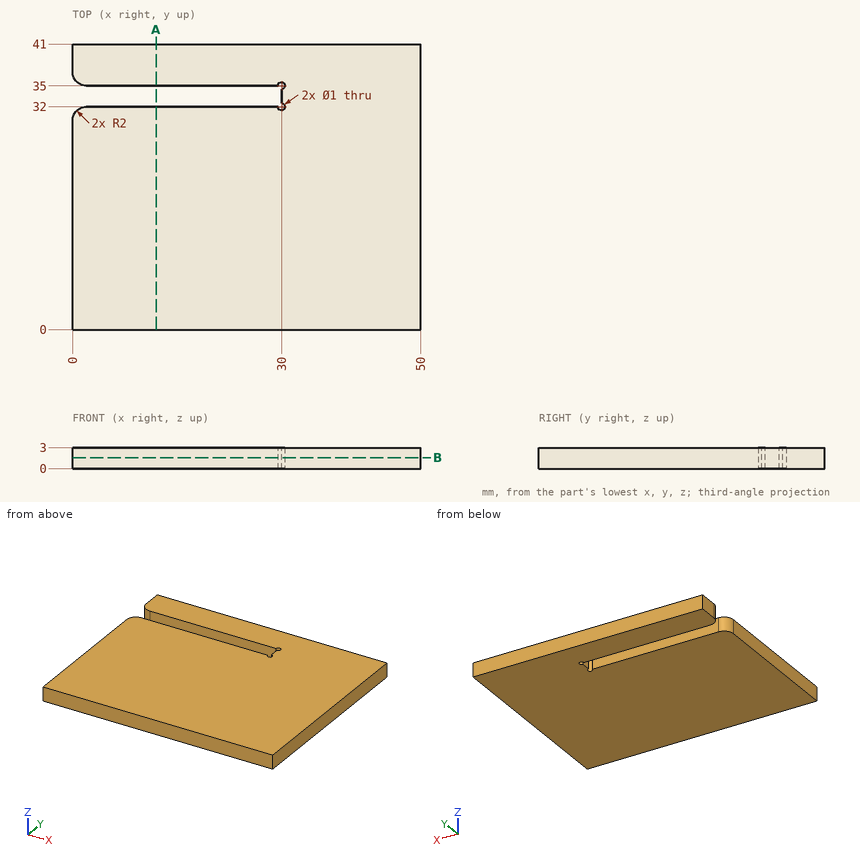
The drawing under review shows one solid part. Ordinate dimensions are in mm from its lowest x, y, z. Coordinates: 2 decimals unless noted, no trailing zeros. Order: outer loops, then holes, each group sorted by start corner. A loop starts at its lowest first (then second) coordinate and runs counter-clockwise, first axis right, second up. Notation, with made-up numbers: M -6.5,28 L 16.5,28 A26 ccw 16.5,56 Z; hole C 69.5,18 d9. An arc over 180 degrees is marked long. Use a Markdown table: item, result.
(1) Wall thickness on probe 1 along Y at (x, z) = (26.5, 2.25): over which ranges is the line inside the solid? List them lowest first.
Worked answers:
| item | result |
|---|---|
| probe 1 | y = 0 to 32, 35 to 41 |
(2) Add section A-A (x = 12). Give the boundary of the cut face in (y, z).
Worked answers:
| item | result |
|---|---|
| outline | M 0,0 L 32,0 L 32,3 L 0,3 Z; M 35,0 L 41,0 L 41,3 L 35,3 Z |
(3) For P1, Ø0.6, axis at y = 33.5, z = 1, coming from the -X side, flat-tipped, find the tip position at first contact; note if it passes through.
Worked answers:
| item | result |
|---|---|
| P1 | stops at x = 30 |
(4) Add section B-B (z = 1.55). Give the boundary of the cut face in (x, y), then the cut area to 3 significant figures.
Worked answers:
| item | result |
|---|---|
| outline | M 0,0 L 50,0 L 50,41 L 0,41 L 0,37 A2 ccw 2,35 L 29.5,35 A0.5 cw long 30,34.5 L 30,32.5 A0.5 cw long 29.5,32 L 2,32 A2 ccw 0,30 Z |
| area | 1,960 mm2 |
